```python
from build123d import *

# Parameters (mm, degrees)
EXTRUDE_1_DEPTH     = 25
SKETCH_2_R          = 1.65
CUT_EXTRUDE_1_DEPTH = 33
SKETCH_3_R          = 1.6
CUT_EXTRUDE_2_DEPTH = 33
CUT_EXTRUDE_3_DEPTH = 14.5


with BuildPart() as part:
    # 草图1 → 凸台-拉伸1 (new body)
    with BuildSketch(Plane.XY):
        Polygon((0, 0), (0, 23.5), (-28, 23.5), (-28, 14.5), (-8, 14.5), (-8, 0), align=None)
    extrude(amount=EXTRUDE_1_DEPTH)

    # 草图2 → 切除-拉伸1 (cut)
    with BuildSketch(Plane(origin=(0, 23.5, 0), x_dir=(1, 0, 0), z_dir=(0, 1, 0))):
        with Locations(Location((-20, -6.5, 0), (0, 0, 180))):
            Circle(SKETCH_2_R)
        with Locations(Location((-20, -18.5, 0), (0, 0, 180))):
            Circle(SKETCH_2_R)
    extrude(amount=-CUT_EXTRUDE_1_DEPTH, mode=Mode.SUBTRACT)

    # 草图3 → 切除-拉伸2 (cut)
    with BuildSketch(Plane.ZY.offset(8)):
        with Locations(Location((6, 11.25, 0), (0, 0, 270))):
            Circle(SKETCH_3_R)
        with Locations(Location((19, 11.25, 0), (0, 0, 270))):
            Circle(SKETCH_3_R)
        with Locations(Location((12.5, 1.8, 0), (0, 0, 270))):
            Circle(SKETCH_3_R)
        with Locations(Location((6, 4.25, 0), (0, 0, 270))):
            Circle(SKETCH_3_R)
        with Locations(Location((19, 4.25, 0), (0, 0, 270))):
            Circle(SKETCH_3_R)
    extrude(amount=-CUT_EXTRUDE_2_DEPTH, mode=Mode.SUBTRACT)

    # 草图4 → 切除-拉伸3 (cut)
    with BuildSketch(Plane.XZ):
        with BuildLine():
            Line((-8, 14.724859546), (-8, 10.275140454))
            ThreePointArc((-8, 10.275140454), (-2.5, 12.5), (-8, 14.724859546))
        make_face()
    extrude(amount=-CUT_EXTRUDE_3_DEPTH, mode=Mode.SUBTRACT)


solid = part.part
```
Geometry: final body of the model. Coordinates: model frame, mm. A direction names the side the tool comes from. Coordinates: 2 decimals unless noted, no trailing zeros. Order: outer loops, then holes, each group sorted by start corner. A loop starts at its lowest first (then second) coordinate and runs counter-clockwise, first axis right, second up. Notation, with made-up numbers: (69, -21.5) -> (87, -21.5) arc R31 cw to (87, 14.5) -> close; hole circle Ø2 at (-28.75, 45.5). An arc over 180 degrees is marked (long way). Write each question's results on one line, items separated by ' | '. Start each with the question number.
1) Cut plane D-D, the plane x = -5.7. Output: boundary loops of the cut face in (y, z).
2) Cut plane A-A, the plane x = -20. Output: boundary loops of the cut face in (y, z).
3) Cut plane C-C, the plane z = 12.5. Output: boundary loops of the cut face in (x, y).
4) Cut plane B-B, the plane y = 4.25. Output: boundary loops of the cut face in (x, z).
5) First-contact query: pin 1 (5 mm diameter, centred on y = 8.5, z = 3.5, fed in from -X); pin 2 (1.9 mm diameter, centred on y = 1.8, z = 12.5, fed in from +X); pin 3 (1.5 mm diameter, centred on x = -13, z = 8, fed in from -Y). Flat tips, straight axial feed; report the tip coordinate or a pass-through.
6) Set-up query: faces 1 (the flat face through (-28, 19, 12)), 2 (the flat face through (-8, 7, 20)), 3 (the cylindrical face through (-2.5, 7.1, 12.4)). Return all of +Z, -Z, +X, -X, +Y, -Y with unobstructed straight access to the full face (end or side cutting, diameter ignored); none if empty.
7) Material intervals for line 1 along Z through (x, y) = (-5.5, 4.25); line 2 along Z through (x, y) = (-2.1, 1.8); line 3 along Z through (x, y) = (-6.5, 4.25), sorted ascending.
8) Mould query, pull axis Z, two halves, no side actions, for faces 4 (the cylindrical face through (-4.06, 12.43, 20.08)), 5 (the flat face through (-2, 0, 12)), 6 (the flat face through (-11, 15, 25)). Classes: released by +Z, released by -Z, zero draft, split by the parting line, or undercut.
Checks:
1) outline: (0, 0) -> (23.5, 0) -> (23.5, 25) -> (0, 25) -> (0, 15.7) -> (14.5, 15.7) -> (14.5, 9.3) -> (0, 9.3) -> close; hole circle Ø3.2 at (4.25, 6); hole circle Ø3.2 at (4.25, 19); hole circle Ø3.2 at (11.25, 6); hole circle Ø3.2 at (11.25, 19)
2) outline: (14.5, 0) -> (23.5, 0) -> (23.5, 4.85) -> (14.5, 4.85) -> close; (14.5, 8.15) -> (23.5, 8.15) -> (23.5, 16.85) -> (14.5, 16.85) -> close; (14.5, 20.15) -> (23.5, 20.15) -> (23.5, 25) -> (14.5, 25) -> close
3) outline: (-28, 14.5) -> (-2.5, 14.5) -> (-2.5, 3.4) -> (0, 3.4) -> (0, 23.5) -> (-28, 23.5) -> close; (-2.5, 0) -> (0, 0) -> (0, 0.2) -> (-2.5, 0.2) -> close
4) outline: (-8, 0) -> (0, 0) -> (0, 4.4) -> (-8, 4.4) -> close; (-8, 7.6) -> (0, 7.6) -> (0, 17.4) -> (-8, 17.4) -> (-8, 14.72) arc R3.2 cw (long way) to (-8, 10.28) -> close; (-8, 20.6) -> (0, 20.6) -> (0, 25) -> (-8, 25) -> close
5) pin 1: x = -8 | pin 2: through | pin 3: y = 14.5
6) face 1: +Z, -Z, -X, +Y, -Y | face 2: +Z, -Z, -X, -Y | face 3: -Y
7) line 1: 0 to 4.4, 7.6 to 9.31, 15.69 to 17.4, 20.6 to 25 | line 2: 0 to 10.9, 14.1 to 25 | line 3: 0 to 4.4, 7.6 to 9.4, 15.6 to 17.4, 20.6 to 25
8) face 4: undercut | face 5: zero draft | face 6: released by +Z
